Geometry: final body of the model. Coordinates: model frame, mm. A direction names the side the tool comes from. Coordinates: 2 decimals unless noted, no trailing zeros. Write each loop counter-clockwise with the first axis right and the second up, starting at its lowest first coordinate (ties: lowest second). Pieces come first, ordered by that corner, then holes.
from build123d import *

# Parameters (mm, degrees)
EXTRUDE_382_DEPTH = 10
FILLET_1302_R     = 0.6


with BuildPart() as part:
    # 草图1 → Extrude 382 (new body)
    with BuildSketch(Plane(origin=(0, 0, 0), x_dir=(0, 0, -1), z_dir=(1, 0, 0))):
        Polygon((12, 6.92820323), (12, -6.92820323), (0, -13.856406461), (-12, -6.92820323), (-12, 6.92820323), (0, 13.856406461), align=None)
    extrude(amount=EXTRUDE_382_DEPTH)

    # 草图2 → 凸台-旋转1 (revolve)
    with BuildSketch(Plane.XY, mode=Mode.PRIVATE) as revolve_1_sk:
        Polygon((0, 0), (75, 0), (75, 6.268), (75, 8), (37, 8), (0, 8), align=None)
    revolve(revolve_1_sk.sketch.rotate(Axis((0, 0, 0), (1, 0, 0)), 90), axis=Axis((0, 0, 0), (1, 0, 0)))

    # 草图3 → 切除-旋转1 (revolve, cut)
    with BuildSketch(Plane.XY):
        Polygon((0, 12), (3.958548116, 18.856406461), (3.958548116, 23.856406461), (-10, 23.856406461), (-10, 12), align=None)
    revolve(axis=Axis((0, 0, 0), (1, 0, 0)), mode=Mode.SUBTRACT)

    # 草图4 → 切除-旋转3 (revolve, cut)
    with BuildSketch(Plane.XY, mode=Mode.PRIVATE) as cut_revolve_3_sk:
        Polygon((10, 11.245), (9.2, 11.706880215), (9.2, 13.856406461), (10, 13.856406461), align=None)
    revolve(cut_revolve_3_sk.sketch.rotate(Axis((0, 0, 0), (1, 0, 0)), 90), axis=Axis((0, 0, 0), (1, 0, 0)), mode=Mode.SUBTRACT)

    # Fillet 1302
    fillet_1302_edges = [part.edges().sort_by_distance(p)[0] for p in [
        (10, 0, -8),
    ]]
    fillet(fillet_1302_edges, radius=FILLET_1302_R)

    # 草图6 → 切除-旋转4 (revolve, cut)
    with BuildSketch(Plane.XY, mode=Mode.PRIVATE) as cut_revolve_4_sk:
        Polygon((74, 8), (76, 8), (75, 6.267949192), align=None)
    revolve(cut_revolve_4_sk.sketch.rotate(Axis((0, 0, 0), (1, 0, 0)), 90), axis=Axis((0, 0, 0), (1, 0, 0)), mode=Mode.SUBTRACT)


solid = part.part
Item 1: Material intervals for probe 1 along X at (y, z) = (5.5, -9); probe 2 along Y at (x, z) = (69, 0.25); probe 3 along Z at (x, y) = (68, -4), sorted ascending.
Derived:
probe 1: x = 0 to 10
probe 2: y = -8 to 8
probe 3: z = -6.93 to 6.93
Item 2: Set-up query: faces 1 (the flat face through (10, -7, 6)), 2 (the conical face through (0.26, 12.45, -0.03)). Return all of +Z, -Z, +X, -X, +Y, -Y with unobstructed straight access to the full face (end or side cutting, diameter ignored); none if empty.
Derived:
face 1: +X
face 2: -X, +Y
Item 3: Section A-A, the plane x = 29. Output: boundary loops of the cut face in (y, z).
Derived:
outline: circle Ø16 at (0, 0)
Item 4: Pin query (flat end, axial travel): pin 1 (4 mm diameter, centred on y = 10.5, z = 1.5, fed in from -X); pin 2 (12 mm diameter, centred on x = 65, z = -4.5, fed in from -Y); pin 3 (4 mm diameter, centred on x = 26.5, y = 6.5, fed in from -Z); pin 4 (1 mm diameter, centred on y = -10, z = 5.5, fed in from +X). Return the tip coordinate at first contact, or that it passes through.
Derived:
pin 1: stops at x = 0
pin 2: stops at y = -8
pin 3: stops at z = -6.61
pin 4: stops at x = 10
